Print and shaded views of the part. All mm, measured from the part's lowest x, y and z. A direction names the side the tool comes from. Give positions to 0.01 mm unless a question says otherwise; leave off trailing zeros. Write each loop counter-clockwise with the first axis right and the second up, starting at its lowest first coordinate (ties: lowest second). Pieces come first, ordered by that corner, then holes. Notation, with made-up numbers: (-33.75, -33) -> (1.25, -33) arc R26 cw to (1.25, -13) -> close; hole circle Ø10 at (-33.75, 85). An arc over 180 degrees is marked (long way). Put each result on its own line as item: value.
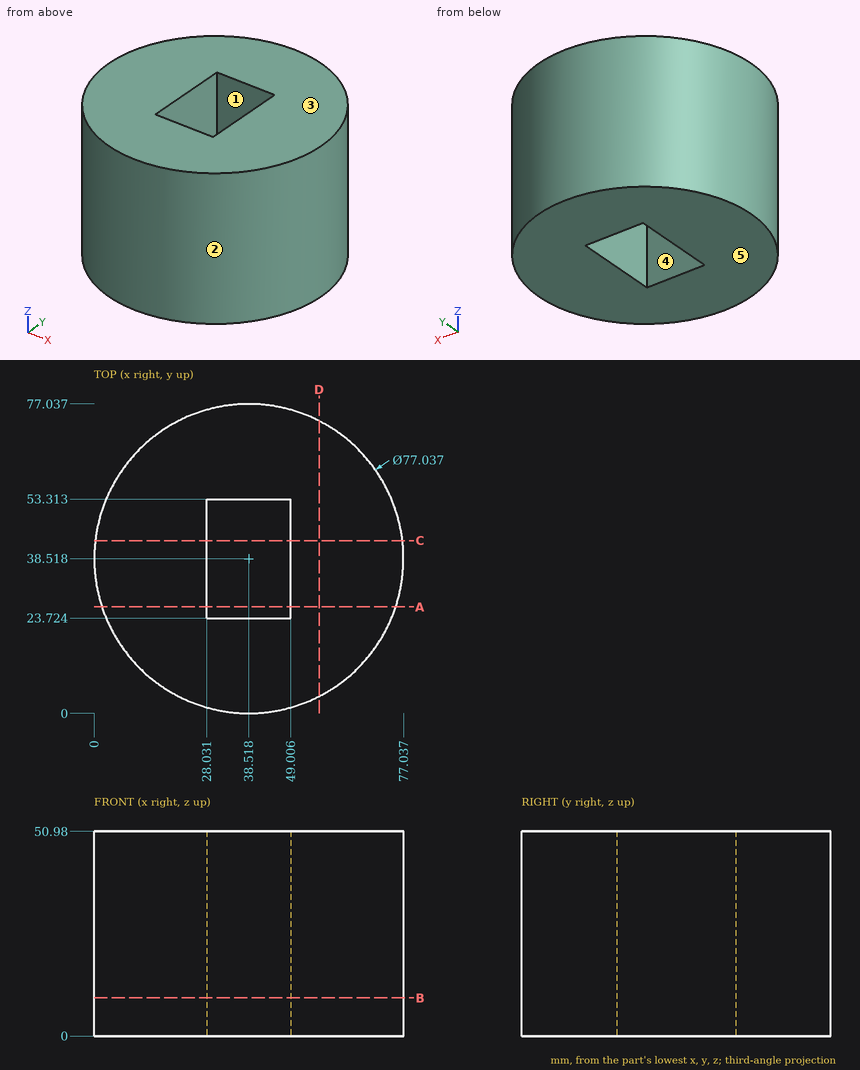
1) Slice it at D-D (x = 56). Write the cut outline in (y, z) (1 decimal), plus the area to 3 significant figures.
Filled sheet:
outline: (4.2, 0) -> (72.8, 0) -> (72.8, 51) -> (4.2, 51) -> close
area: 3,500 mm2
2) Slice it at A-A (y = 26.5). Write the cut outline in (x, z) (1 decimal), plus the area to 3 significant figures.
Filled sheet:
outline: (1.9, 0) -> (28, 0) -> (28, 51) -> (1.9, 51) -> close; (49, 0) -> (75.1, 0) -> (75.1, 51) -> (49, 51) -> close
area: 2,660 mm2
3) Slice it at B-B (z = 9.5). Write the cut outline in (x, y) (1 decimal).
Filled sheet:
outline: circle Ø77 at (38.5, 38.5); hole (28, 23.7) -> (49, 23.7) -> (49, 53.3) -> (28, 53.3) -> close
4) Tool access for the marked faces 4 and 5: list every direction of +Z, -Z, +X, -X, +Y, -Y with a clear straight run to the whole face (end or side of a thin tool).
Filled sheet:
face 4: +Z, -Z
face 5: -Z, +X, -X, +Y, -Y
5) Pin check, flat tips, straight feed: pin 1 (1.5 mm diameter, centred on x = 13, z = 43, fed in from -Y); pin 2 (1 mm diameter, centred on y = 51, z = 32, fed in from +X) (1 decimal); pin 3 (10 mm diameter, centred on y = 58.5, z = 43.5, fed in from -X). Stop position of each tip, or through.
Filled sheet:
pin 1: y = 9.02
pin 2: x = 75.1
pin 3: x = 3.03
6) Slice it at C-C (y = 43). Write the cut outline in (x, z) (1 decimal), plus the area to 3 significant figures.
Filled sheet:
outline: (0.3, 0) -> (28, 0) -> (28, 51) -> (0.3, 51) -> close; (49, 0) -> (76.8, 0) -> (76.8, 51) -> (49, 51) -> close
area: 2,830 mm2
7) Wall check: L1, parallel to Y at x = 38, z = 34.5; L2, parallel to X at y = 26.5, z = 39 (1 decimal); L3, parallel to X at y = 51.5, z = 17 (1 decimal). Give the ranges that are in metal, low to high.
Filled sheet:
L1: 0 to 23.72, 53.31 to 77.03
L2: 1.9 to 28, 49 to 75.1
L3: 2.3 to 28, 49 to 74.8
8) Pull direction X, two halves, no side cores. Call the marked faces 1, 2 and 3: released by +X, released by -X, zero draft, split by the parting line, or undercut.
Filled sheet:
face 1: undercut
face 2: split by the parting line
face 3: zero draft
